Input: part model. Units: mm. Frame: model coordinates. A direction names the side the tool comes from. Round coordinates to 2 decimals unless told otherwise and drop trailing zeros. Loops run counter-clockwise (first coordinate to the right, second up) from the corner with the lowest first, then second, coordinate; pieces in that order, holes last. Notation, with made-up numbers: M -35,56.5 L -24,56.5 A17 cw -24,83.5 Z; hole C 80.5,78 d11. An arc over 180 degrees is marked long. Return JSON: item names as keys, results as strings. Group by question number.
1) Contact query for flat-ended pins moving along their axis: P1, Ø5, axis at y = 13.5, z = -3, coming from the -X side; P2, Ø3, axis at x = 16, z = 0, coming from the +Y side; P3, Ø1, axis at y = 14.5, z = 3.5, coming from the +X side. Output: stop coordinate, or through.
2) Material intervals for line 1 (X direction, y = 9.5, z = -1.75); line 2 (X direction, y = 1.7, z = 0); line 3 (X direction, y = 1.65, z = 0), sorted ascending. Write a range as from..to.
3) Section C-C (z = -4). Output: boundary loops of the cut face in (x, y).
4) Section D-D (y = 13.5). Output: boundary loops of the cut face in (x, z).
5) Mould query, pull axis Y, two halves, no side actions, for faces 4 (the face through (-11.289, 4.804, -0.07)), 5 (the face through (29, 10, 0)), 6 (the face through (32.196, 1.711, -0.07)), 7 (the face through (-18, 9, 0)). Classes: +Y half, -Y half, draft (parallel to the pull), parting line (faces both ways), or undercut.
6) Access query for faces 1 (the face through (-16.9, 15.46, -0.07)), 2 (the face through (-12.463, 13.01, -0.07)), 3 (the face through (8, 3, 0)). Directions: +Z, -Z, +X, -X, +Y, -Y. A direction counts if a zero-diameter tool reaches every point of the face in a straight line with its end or side. Return the directions, or none.
7) Section A-A (z = 0). Output: boundary loops of the cut face in (x, y).
8) Section B-B (x = 0). Output: boundary loops of the cut face in (y, z).
from build123d import *

# Parameters (mm, degrees)
SKETCH1_W           = 42
SKETCH1_H           = 10
SKETCH1_R           = 1.25
BOSS_EXTRUDE1_DEPTH = 3
SKETCH2_W           = 5
SKETCH2_H           = 10
BOSS_EXTRUDE2_DEPTH = 18
SKETCH3_W           = 10
SKETCH3_H           = 3
BOSS_EXTRUDE3_DEPTH = 2
SKETCH4_W           = 10
SKETCH4_H           = 3
BOSS_EXTRUDE4_DEPTH = 2
FILLET1_R           = 6


with BuildPart() as part:
    # Sketch1 → Boss-Extrude1 (new body)
    with BuildSketch(Plane(origin=(0, 0, 0), x_dir=(1, 0, 0), z_dir=(0, 1, 0))):
        with Locations((8, 0)):
            Rectangle(SKETCH1_W, SKETCH1_H)
        with Locations(Location((0, 0, 0), (0, 0, 270))):
            Circle(SKETCH1_R, mode=Mode.SUBTRACT)
        with Locations(Location((16, 0, 0), (0, 0, 270))):
            Circle(SKETCH1_R, mode=Mode.SUBTRACT)
    extrude(amount=BOSS_EXTRUDE1_DEPTH)

    # Sketch2 → Boss-Extrude2 (add)
    with BuildSketch(Plane.XZ):
        with Locations((-15.5, 0)):
            Rectangle(SKETCH2_W, SKETCH2_H)
        with Locations((31.5, 0)):
            Rectangle(SKETCH2_W, SKETCH2_H)
    extrude(amount=-BOSS_EXTRUDE2_DEPTH)

    # Sketch3 → Boss-Extrude3 (add)
    with BuildSketch(Plane(origin=(-13, 0, 0), x_dir=(0, 0, -1), z_dir=(1, 0, 0))):
        with Locations((0, 16.5)):
            Rectangle(SKETCH3_W, SKETCH3_H)
    extrude(amount=BOSS_EXTRUDE3_DEPTH)

    # Sketch4 → Boss-Extrude4 (add)
    with BuildSketch(Plane.ZY.offset(-29)):
        with Locations((0, 16.5)):
            Rectangle(SKETCH4_W, SKETCH4_H)
    extrude(amount=BOSS_EXTRUDE4_DEPTH)

    # Fillet1
    # the kernel refuses this fillet: 6 mm, written as the material it adds along each edge
    with BuildSketch(Plane(origin=(29, 15, 5), x_dir=(-1, 0, 0), z_dir=(0, 0, -1))) as fillet1_piece_1:
        with BuildLine():
            CenterArc((6, -4.472135955), FILLET1_R, 131.810314896, 48.189685104)
            Line((0, -4.472135955), (-0.12, -4.472135955))
            Line((-0.12, -4.472135955), (-0.12, 0))
            Line((-0.12, 0), (0, 0.12))
            ThreePointArc((0, 0.12), (1, 0.12), (1.92, 0.089442719))
            Line((1.92, 0.089442719), (2, 0))
        make_face()
    extrude(amount=10)
    with BuildSketch(Plane(origin=(29, 3, 5), x_dir=(0, 1, 0), z_dir=(0, 0, -1))) as fillet1_piece_2:
        with BuildLine():
            CenterArc((FILLET1_R, -FILLET1_R), FILLET1_R, 90, 90)
            Line((0, -FILLET1_R), (-FILLET1_R * 0.02, -FILLET1_R))
            Line((-FILLET1_R * 0.02, -FILLET1_R), (-FILLET1_R * 0.02, FILLET1_R * 0.02))
            Line((-FILLET1_R * 0.02, FILLET1_R * 0.02), (FILLET1_R, FILLET1_R * 0.02))
            Line((FILLET1_R, FILLET1_R * 0.02), (FILLET1_R, 0))
        make_face()
    extrude(amount=10)
    with BuildSketch(Plane(origin=(-13, 15, -5), x_dir=(0, -1, 0), z_dir=(0, 0, 1))) as fillet1_piece_3:
        with BuildLine():
            CenterArc((4.472135955, 6), FILLET1_R, 221.810314896, 48.189685104)
            Line((0, 2), (-0.089442719, 1.92))
            ThreePointArc((-0.089442719, 1.92), (-0.12, 1), (-0.12, 0))
            Line((-0.12, 0), (0, -0.12))
            Line((0, -0.12), (4.472135955, -0.12))
            Line((4.472135955, -0.12), (4.472135955, 0))
        make_face()
    extrude(amount=10)
    with BuildSketch(Plane(origin=(-13, 3, -5), x_dir=(1, 0, 0), z_dir=(0, 0, 1))) as fillet1_piece_4:
        with BuildLine():
            CenterArc((FILLET1_R, FILLET1_R), FILLET1_R, 180, 90)
            Line((0, FILLET1_R), (-FILLET1_R * 0.02, FILLET1_R))
            Line((-FILLET1_R * 0.02, FILLET1_R), (-FILLET1_R * 0.02, -FILLET1_R * 0.02))
            Line((-FILLET1_R * 0.02, -FILLET1_R * 0.02), (FILLET1_R, -FILLET1_R * 0.02))
            Line((FILLET1_R, -FILLET1_R * 0.02), (FILLET1_R, 0))
        make_face()
    extrude(amount=10)
    # the kernel refuses this fillet: 6 mm, written as the material it takes off along each edge
    with BuildSketch(Plane(origin=(-18, 0, -20), x_dir=(1, 0, 0), z_dir=(0, 0, 1))) as fillet1_2_piece_1:
        with BuildLine():
            CenterArc((FILLET1_R, FILLET1_R), FILLET1_R, 180, 90)
            Line((0, FILLET1_R), (-FILLET1_R * 0.02, FILLET1_R))
            Line((-FILLET1_R * 0.02, FILLET1_R), (-FILLET1_R * 0.02, -FILLET1_R * 0.02))
            Line((-FILLET1_R * 0.02, -FILLET1_R * 0.02), (FILLET1_R, -FILLET1_R * 0.02))
            Line((FILLET1_R, -FILLET1_R * 0.02), (FILLET1_R, 0))
        make_face()
    extrude(amount=40, mode=Mode.SUBTRACT)
    with BuildSketch(Plane(origin=(-18, 18, -20), x_dir=(1, 0, 0), z_dir=(0, 0, 1)), Plane(origin=(34, 0, -20), x_dir=(-1, 0, 0), z_dir=(0, 0, 1)), Plane(origin=(34, 18, -20), x_dir=(0, -1, 0), z_dir=(0, 0, 1))) as fillet1_2_piece_2:
        with BuildLine():
            CenterArc((FILLET1_R, -FILLET1_R), FILLET1_R, 90, 90)
            Line((0, -FILLET1_R), (-FILLET1_R * 0.02, -FILLET1_R))
            Line((-FILLET1_R * 0.02, -FILLET1_R), (-FILLET1_R * 0.02, FILLET1_R * 0.02))
            Line((-FILLET1_R * 0.02, FILLET1_R * 0.02), (FILLET1_R, FILLET1_R * 0.02))
            Line((FILLET1_R, FILLET1_R * 0.02), (FILLET1_R, 0))
        make_face()
    extrude(amount=40, mode=Mode.SUBTRACT)
    with BuildSketch(Plane(origin=(27, 18, -17.990381057), x_dir=(1, 0, 0), z_dir=(0, 0, 1))) as fillet1_2_piece_3:
        with BuildLine():
            CenterArc((5.196152423, -6), FILLET1_R, 90, 60)
            Line((0, -3), (-0.103923048, -2.94))
            ThreePointArc((-0.103923048, -2.94), (-0.12, -1.5), (-0.12, 0))
            Line((-0.12, 0), (0, 0.12))
            Line((0, 0.12), (5.196152423, 0.12))
            Line((5.196152423, 0.12), (5.196152423, 0))
        make_face()
    extrude(amount=35.980762114, mode=Mode.SUBTRACT)
    with BuildSketch(Plane(origin=(-11, 18, 17.990381057), x_dir=(0, -1, 0), z_dir=(0, 0, -1))) as fillet1_2_piece_4:
        with BuildLine():
            CenterArc((6, 5.196152423), FILLET1_R, 180, 60)
            Line((0, 5.196152423), (-0.12, 5.196152423))
            Line((-0.12, 5.196152423), (-0.12, 0))
            Line((-0.12, 0), (0, -0.12))
            ThreePointArc((0, -0.12), (1.5, -0.12), (2.94, -0.103923048))
            Line((2.94, -0.103923048), (3, 0))
        make_face()
    extrude(amount=35.980762114, mode=Mode.SUBTRACT)


solid = part.part
Returned:
{
 "1": {"P1": "stops at x = -18", "P2": "stops at y = 3", "P3": "stops at x = 33.66"},
 "2": {"line 1": "x = -18..-13, 29..34", "line 2": "x = -16.18..-1.25, 1.25..14.75, 17.25..32.18", "line 3": "x = -16.13..-1.25, 1.25..14.75, 17.25..32.13"},
 "3": {"outline": "M -18,6 A6 ccw -12,0 L 28,0 A6 ccw 34,6 L 34,12 A6 ccw 30.1,17.62 A6 ccw 27,15 A6 cw 29,10.53 L 29,9 A6 cw 23,3 L -7,3 A6 cw -13,9 L -13,10.53 A6 cw -11,15 A6 ccw -14.1,17.62 A6 ccw -18,12 Z"},
 "4": {"outline": "M -17.81,-5 L -12.21,-5 L -12.21,5 L -17.81,5 Z; M 28.21,-5 L 33.81,-5 L 33.81,5 L 28.21,5 Z"},
 "5": {"face 4": "undercut", "face 5": "undercut", "face 6": "-Y half", "face 7": "draft"},
 "6": {"face 1": "+Z, -Z, -X, +Y", "face 2": "+Z, -Z", "face 3": "+Z, -Z, +Y"},
 "7": {"outline": "M -18,6 A6 ccw -12,0 L -1.25,0 L -1.25,3 L -7,3 A6 cw -13,9 L -13,10.53 A6 cw -11,15 A6 ccw -14.1,17.62 A6 ccw -18,12 Z; M 1.25,0 L 14.75,0 L 14.75,3 L 1.25,3 Z; M 17.25,0 L 28,0 A6 ccw 34,6 L 34,12 A6 ccw 30.1,17.62 A6 ccw 27,15 A6 cw 29,10.53 L 29,9 A6 cw 23,3 L 17.25,3 Z"},
 "8": {"outline": "M 0,-5 L 3,-5 L 3,-1.25 L 0,-1.25 Z; M 0,1.25 L 3,1.25 L 3,5 L 0,5 Z"}
}
